Part model, mm, in its own coordinate system. Coordinates: 2 decimals unless noted, no trailing zeros. Loops run counter-clockwise (first coordinate to the right, second up) from the corner with the lowest first, then second, coordinate; pieces in that order, holes last. Notation, with made-up numbers: (59, 37) - (75, 37) arc R21 cw to (75, 49) - close; hole circle Ø5 at (79, 76). An arc over 180 degrees is marked (long way). Answer as CSV lines item,"result".
from build123d import *

# Parameters (mm, degrees)
SKETCH_1_R          = 50
SKETCH_1_R_2        = 47.5
CUT_EXTRUDE_1_DEPTH = 150
SKETCH_3_R          = 50
SKETCH_3_R_2        = 47.5
EXTRUDE_1_DEPTH     = 350
SKETCH_5_R          = 50
SKETCH_5_R_2        = 47.5


with BuildPart() as part:
    # 草图1 → 旋转1 (revolve)
    with BuildSketch(Plane.XY, mode=Mode.PRIVATE) as revolve_1_sk:
        with Locations((250, 0)):
            Circle(SKETCH_1_R)
        with Locations((250, 0)):
            Circle(SKETCH_1_R_2, mode=Mode.SUBTRACT)
    revolve(revolve_1_sk.sketch.rotate(Axis((0, 0, 0), (0, 1, 0)), 90), axis=Axis((0, 0, 0), (0, 1, 0)))

    # 草图2 → 切除-拉伸1 (cut, symmetric)
    with BuildSketch(Plane(origin=(0, 0, 0), x_dir=(1, 0, 0), z_dir=(0, 1, 0))):
        Polygon((-384.261644324, 0), (443.109902211, 0), (321.917450325, -325.996042455), (-266.565128549, -318.421514212), align=None)
    extrude(amount=CUT_EXTRUDE_1_DEPTH, both=True, mode=Mode.SUBTRACT)

    # 草图3 → 凸台-拉伸1 (add)
    with BuildSketch(Plane.XY):
        with Locations((250, 0)):
            Circle(SKETCH_3_R)
        with Locations((250, 0)):
            Circle(SKETCH_3_R_2, mode=Mode.SUBTRACT)
    extrude_1 = extrude(amount=EXTRUDE_1_DEPTH)

    # 镜向1: 凸台-拉伸1 across plane
    add(extrude_1.mirror(Plane(origin=(0, 0, 0), x_dir=(0, 0, 1), z_dir=(1, 0, 0))))

    # 扫描1: sweep along a path in 草图4
    with BuildLine(Plane(origin=(0, 0, 0), x_dir=(1, 0, 0), z_dir=(0, 1, 0))) as sweep_1_path:
        Line((250, -350), (250, -450))
        Line((250, -450), (0, -450))
    # 草图5 → 扫描1 (sweep)
    with BuildSketch(Plane.XY.offset(350)):
        with Locations((250, 0)):
            Circle(SKETCH_5_R)
        with Locations((250, 0)):
            Circle(SKETCH_5_R_2, mode=Mode.SUBTRACT)
    sweep_1 = sweep(path=sweep_1_path.line, transition=Transition.RIGHT)

    # 镜向2: 扫描1 across plane
    add(sweep_1.mirror(Plane(origin=(0, 0, 0), x_dir=(0, 0, 1), z_dir=(1, 0, 0))))


solid = part.part
Q1. Saw through at D-D (x = -61.5). Count the separate pieces of the cut face and the enclosed holes in it, then the cut area to 3 significant figures.
Results:
separate pieces,"2"
enclosed holes,"2"
area,"1,560 mm^2"
Q2. Wall check: L1, parallel to X at y = -3, z = 295.5; L2, parallel to X at y = 0, z = 390; L3, parallel to Y at x = -212, z = 450. Give the ranges that are in metal, low to high.
Results:
L1,"x = -299.91 to -297.41, -202.59 to -200.09, 200.09 to 202.59, 297.41 to 299.91"
L2,"x = -300 to -297.5, -202.5 to -200, 200 to 202.5, 297.5 to 300"
L3,"y = -50 to -47.5, 47.5 to 50"
Q3. Saw through at B-B (z = 450). Give the cut face in (x, y), then the cut area to 3 significant figures.
Results:
outline,"(-250, -50) - (250, -50) arc R50 ccw to (250, 50) - (-250, 50) arc R50 ccw to start; hole (-250, -47.5) - (250, -47.5) arc R47.5 ccw to (250, 47.5) - (-250, 47.5) arc R47.5 ccw to start"
area,"3,270 mm^2"
Q4. Saw through at A-A (y = 0). Give the cut face in (x, z), then the cut area to 3 significant figures.
Results:
outline,"(-300, 0) arc R300 ccw to (300, 0) - (300, 500) - (-300, 500) - close; (-202.5, 0) arc R202.5 ccw to (202.5, 0) - (202.5, 402.5) - (-202.5, 402.5) - close; hole (-297.5, 0) arc R297.5 ccw to (297.5, 0) - (297.5, 497.5) - (-297.5, 497.5) - close; hole (-200, 0) arc R200 ccw to (200, 0) - (200, 400) - (-200, 400) - close"
area,"10,900 mm^2"
Q5. Flat gauge pins, fed straight in: pin 1 (6 mm diameter, centred on y = -17, z = -8.5, fed in from +X); pin 2 (5 mm diameter, centred on x = -193, y = 22, fed in from -Z); pin 3 (12 mm diameter, centred on y = 22.5, z = 307, fed in from -X). Where does each tip first touch, or does it go through?
Results:
pin 1,"stops at x = 297.88"
pin 2,"stops at z = -225.61"
pin 3,"stops at x = -297.2"
Q6. Saw through at C-C (z = 21). Give the cut face in (x, y).
Results:
outline,"circle Ø100 at (-250, 0); circle Ø100 at (250, 0); hole circle Ø95 at (-250, 0); hole circle Ø95 at (250, 0)"
